Source: CAD feature listing. Evaluate the final solid. Frame: model axes, mm. Face numbers are marked on the shaded views. A direction names the side the tool comes from. Round coordinates to 2 decimals unless told otherwise and drop trailing zeros. Write each loop counter-clockwise with the first axis right and the second up, starting at its lowest first coordinate (ties: lowest second). Pieces come first, ordered by that corner, then holes. Notation, with made-up numbers: M 13,34.25 L 59,34.25 A23 ccw 59,73.25 Z; hole C 37.5,-21 d10. An arc over 180 degrees is marked long. Answer in a Markdown table with one row per item.
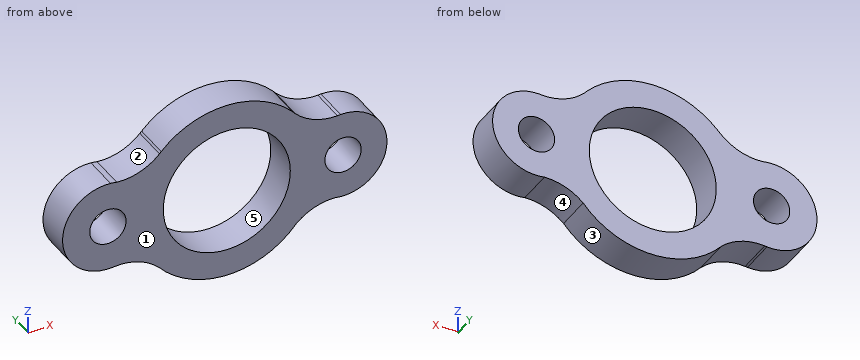
from build123d import *

# Parameters (mm, degrees)
F0_R     = 12.7
F0_R_2   = 44.45
F1_DEPTH = 25.4


with BuildPart() as f1:
    # F0 (on Front) → F1 (new body)
    with BuildSketch(Plane.XZ):
        with BuildLine():
            ThreePointArc((-78.322921, -31.378096), (-61.741608, -33.273322), (-47.561115, -42.07363))
            ThreePointArc((-47.561115, -42.07363), (0.884923, -63.493834), (48.715187, -40.731813))
            ThreePointArc((48.715187, -40.731813), (61.225405, -32.799779), (75.815182, -30.23831))
            ThreePointArc((75.815182, -30.23831), (112.047103, -1.913109), (79.61425, 30.693318))
            ThreePointArc((79.61425, 30.693318), (78.511328, 30.574208), (77.405407, 30.487258))
            ThreePointArc((77.405407, 30.487258), (61.368574, 32.920927), (47.797419, 41.804985))
            ThreePointArc((47.797419, 41.804985), (46.84664, 42.808286), (45.932881, 43.845416))
            ThreePointArc((45.932881, 43.845416), (0.021282, 63.499996), (-45.903481, 43.876194))
            ThreePointArc((-45.903481, 43.876194), (-46.498842, 43.220557), (-47.109281, 42.578934))
            ThreePointArc((-47.109281, 42.578934), (-60.807213, 33.568892), (-77.023302, 31.149665))
            ThreePointArc((-77.023302, 31.149665), (-79.194575, 31.361818), (-81.350145, 31.6979))
            ThreePointArc((-81.350145, 31.6979), (-114.910072, -0.722366), (-79.91004, -31.582373))
            ThreePointArc((-79.91004, -31.582373), (-79.117553, -31.471901), (-78.322921, -31.378096))
        make_face()
        with Locations((-83.168291, 0)):
            Circle(F0_R, mode=Mode.SUBTRACT)
        Circle(F0_R_2, mode=Mode.SUBTRACT)
        with Locations((81.363559, 0)):
            Circle(F0_R, mode=Mode.SUBTRACT)
        with BuildLine():
            ThreePointArc((-79.91004, -31.582373), (-79.115193, -31.490235), (-78.322921, -31.378096))
            ThreePointArc((-78.322921, -31.378096), (-79.117553, -31.471901), (-79.91004, -31.582373))
        make_face()
        with BuildLine():
            ThreePointArc((77.405407, 30.487258), (78.511328, 30.574208), (79.61425, 30.693318))
            ThreePointArc((79.61425, 30.693318), (78.507969, 30.610219), (77.405407, 30.487258))
        make_face()
        with BuildLine():
            ThreePointArc((-77.023302, 31.149665), (-79.177299, 31.498166), (-81.350145, 31.6979))
            ThreePointArc((-81.350145, 31.6979), (-79.194575, 31.361818), (-77.023302, 31.149665))
        make_face()
        with BuildLine():
            ThreePointArc((45.932881, 43.845416), (46.84664, 42.808286), (47.797419, 41.804985))
            ThreePointArc((47.797419, 41.804985), (46.876253, 42.835346), (45.932881, 43.845416))
        make_face()
        with BuildLine():
            ThreePointArc((-45.903481, 43.876194), (-46.510904, 43.231768), (-47.109281, 42.578934))
            ThreePointArc((-47.109281, 42.578934), (-46.498842, 43.220557), (-45.903481, 43.876194))
        make_face()
    extrude(amount=F1_DEPTH)


solid = f1.part
Q1. Section B-B (z = 0). Return loops of the section in (x, y).
Solutions:
| item | result |
|---|---|
| outline | M -114.92,-25.4 L -95.87,-25.4 L -95.87,0 L -114.92,0 Z; M -70.47,-25.4 L -44.45,-25.4 L -44.45,0 L -70.47,0 Z; M 44.45,-25.4 L 68.66,-25.4 L 68.66,0 L 44.45,0 Z; M 94.06,-25.4 L 112.11,-25.4 L 112.11,0 L 94.06,0 Z |
Q2. Access query for the marked faces 4 and 5. Directions: +Z, -Z, +X, -X, +Y, -Y. A direction counts if a zero-diameter tool reaches every point of the face in a straight line with its end or side. Return the directions, or none.
Solutions:
| item | result |
|---|---|
| face 4 | -Z, +Y, -Y |
| face 5 | +Y, -Y |
Q3. Section C-C (z = 18). Return loops of the section in (x, y).
Solutions:
| item | result |
|---|---|
| outline | M -109.32,-25.4 L -40.64,-25.4 L -40.64,0 L -109.32,0 Z; M 40.64,-25.4 L 106.29,-25.4 L 106.29,0 L 40.64,0 Z |
Q4. Material intervals for probe 1 along Z at (x, y) = (0, -12.25); probe 2 along Z at (x, y) = (92, -16); probe 3 along X at (y, z) = (-8, -4), sorted ascending.
Solutions:
| item | result |
|---|---|
| probe 1 | z = -63.5 to -44.45, 44.45 to 63.5 |
| probe 2 | z = -28.84 to -6.94, 6.94 to 28.84 |
| probe 3 | x = -114.67 to -95.22, -71.11 to -44.27, 44.27 to 69.31, 93.42 to 111.85 |
Q5. Pull-direction query (X, two-part tool) for the marked faces 1, 2 and 3; classes: pulls with the +X half, pulls with the -X half, needs draft (parallel to the pull), parting line crosses it, or undercut.
Solutions:
| item | result |
|---|---|
| face 1 | needs draft |
| face 2 | undercut |
| face 3 | parting line crosses it |
Q6. Contact query for flat-ended pins moving along their axis: pin 1 Ø6 at (x, y) = (7.5, -15) entering from -Z; pin 2 Ø6 at (x, y) = (-13.5, -18) entering from +Z; pin 3 Ø10 at (y, z) = (-7.5, 33.5) entering from +X. Output: stop coordinate, or through.
Solutions:
| item | result |
|---|---|
| pin 1 | stops at z = -63.34 |
| pin 2 | stops at z = 62.63 |
| pin 3 | stops at x = 92.89 |
Q7. Section D-D (y = -9). Return loops of the section in (x, z).
Solutions:
| item | result |
|---|---|
| outline | M -81.35,31.7 A31.75 ccw long -79.91,-31.58 A31.75 ccw -78.32,-31.38 A38.1 cw -47.56,-42.07 A63.5 ccw 48.72,-40.73 A38.1 cw 75.82,-30.24 A30.74 ccw long 79.61,30.69 A30.74 ccw 77.41,30.49 A38.1 cw 47.8,41.8 A63.5 ccw 45.93,43.85 A63.5 ccw -45.9,43.88 A63.5 ccw -47.11,42.58 A38.1 cw -77.02,31.15 A31.75 ccw Z; hole C -83.17,0 d25.4; hole C 0,0 d88.9; hole C 81.36,0 d25.4 |
Q8. Section A-A (x = 0). Return loops of the section in (y, z).
Solutions:
| item | result |
|---|---|
| outline | M -25.4,-63.5 L 0,-63.5 L 0,-44.45 L -25.4,-44.45 Z; M -25.4,44.45 L 0,44.45 L 0,63.5 L -25.4,63.5 Z |
